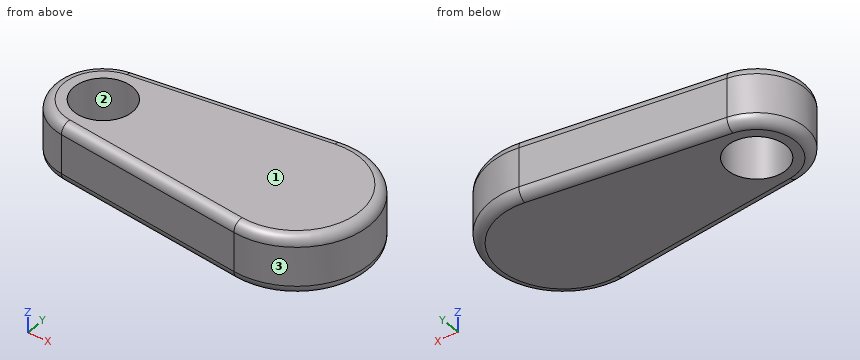
from build123d import *

# Parameters (mm, degrees)
F1_DEPTH = 12
F2_R     = 6
F3_DEPTH = 12
F4_R     = 2


with BuildPart() as f1:
    # F0 (on Top) → F1 (new body)
    with BuildSketch(Plane.XY):
        with BuildLine():
            Line((38.125, 14.882351), (-1.25, 9.921567))
            ThreePointArc((-1.25, 9.921567), (-10, 0), (-1.25, -9.921567))
            Line((-1.25, -9.921567), (38.125, -14.882351))
            ThreePointArc((38.125, -14.882351), (55, 0), (38.125, 14.882351))
        make_face()
    extrude(amount=F1_DEPTH)

    # F2 (on face) → F3 (cut, through all)
    with BuildSketch(Plane.XY.offset(12)):
        Circle(F2_R)
    extrude(amount=-F3_DEPTH, mode=Mode.SUBTRACT)

    # F4
    f4_edges = [f1.edges().sort_by_distance(p)[0] for p in [
        (18.4375, 12.401959, 12),
        (18.4375, 12.401959, 0),
    ]]
    fillet(f4_edges, radius=F4_R)


solid = f1.part
The model under review builds one solid part; all positions refer to its coordinate system, in mm. Face numbers are marked on the shaded views. Coordinates: 2 decimals unless noted, no trailing zeros. Write each loop counter-clockwise with the first axis right and the second up, starting at its lowest first coordinate (ties: lowest second). Pieces come first, ordered by that corner, then holes. Notation, with made-up numbers: M 25.25,23.25 L 35.25,23.25 A29 cw 35.25,60.25 Z; hole C -32.5,72 d10. An arc over 180 degrees is marked long. Put each result on its own line as item: value.
1) Clearance check with flat-ended pins moving along their axes: pin 1 Ø5 at (x, z) = (8, 7.5) entering from +Y; pin 2 Ø5 at (y, z) = (-9.5, 7) entering from +X; pin 3 Ø4 at (y, z) = (-5, 7) entering from -X. State where each tip first meets the part, or that it passes through.
Computed:
pin 1: stops at y = 11.4
pin 2: stops at x = 53.27
pin 3: stops at x = -9.54
2) Wall thickness on probe 1 along Y at (x, z) = (0, 3.25); probe 2 along X at (y, z) = (-1, 6.75); probe 3 along X at (y, z) = (-2.25, 9.25): over which ranges is each line inside the solid? List them lowest first. Write a range as [from, to].
Computed:
probe 1: y = [-10.08, -6], [6, 10.08]
probe 2: x = [-9.95, -5.92], [5.92, 54.97]
probe 3: x = [-9.74, -5.56], [5.56, 54.83]
3) Draft analysis for pull direction Y (two halves, no side actions). For the marked faces 1, 2 and 3, state which applies: released by +Y, released by -Y, zero draft, split by the parting line, or undercut.
Computed:
face 1: zero draft
face 2: undercut
face 3: split by the parting line
4) Add section A-A on y = 0. Give the boundary of the cut face in (x, z), then the cut area to 3 significant figures.
Computed:
outline: M -10,2 A2 ccw -8,0 L -6,0 L -6,12 L -8,12 A2 ccw -10,10 Z; M 6,0 L 53,0 A2 ccw 55,2 L 55,10 A2 ccw 53,12 L 6,12 Z
area: 633 mm2
5) Add section B-B on z = 7. Give the boundary of the cut face in (x, y) (3 decimals), then the cut area to 3 significant figures.
Computed:
outline: M -1.25,-9.922 L 38.125,-14.882 A15 ccw long 38.125,14.882 L -1.25,9.922 A10 ccw Z; hole C 0,0 d12
area: 1,410 mm2
